Part model, mm, in its own coordinate system. A direction names the side the tool comes from. Give positions to 0.01 mm unless a question says otherwise; leave off trailing zeros. Write each loop counter-clockwise with the first axis right and the second up, starting at its lowest first coordinate (ties: lowest second). Pieces come first, ordered by that corner, then holes.
```python
from build123d import *

# Parameters (mm, degrees)
EXTRUDE_1_DEPTH     = 20
SKETCH_2_R          = 1.25
EXTRUDE_2_DEPTH     = 6
SKETCH_3_R          = 1.25
CUT_EXTRUDE_1_DEPTH = 6


with BuildPart() as part:
    # 草图1 → 凸台-拉伸1 (new body)
    with BuildSketch(Plane(origin=(0, 0, 0), x_dir=(1, 0, 0), z_dir=(0, 1, 0))):
        Polygon((2.125123473, -1.583145674), (2.433606108, 1.048838076), (0.308482635, 2.631983751), (-2.125123473, 1.583145674), (-2.433606108, -1.048838076), (-0.308482635, -2.631983751), align=None)
    extrude(amount=EXTRUDE_1_DEPTH)

    # 草图2 → 凸台-拉伸2 (add)
    with BuildSketch(Plane(origin=(0, 20, 0), x_dir=(1, 0, 0), z_dir=(0, 1, 0))):
        Circle(SKETCH_2_R)
    extrude(amount=EXTRUDE_2_DEPTH)

    # 草图3 → 切除-拉伸1 (cut)
    with BuildSketch(Plane.XZ):
        Circle(SKETCH_3_R)
    extrude(amount=-CUT_EXTRUDE_1_DEPTH, mode=Mode.SUBTRACT)


solid = part.part
```
1) Saw through at D-D, the plane z = 0. Write the cut outline in (x, y).
Answers follow:
outline: (-2.31, 0) - (-1.25, 0) - (-1.25, 6) - (1.25, 6) - (1.25, 0) - (2.31, 0) - (2.31, 20) - (1.25, 20) - (1.25, 26) - (-1.25, 26) - (-1.25, 20) - (-2.31, 20) - close
2) Saw through at A-A, the plane y = 3. Write the cut outline in (x, z), then the cut area to 3 significant figures.
Answers follow:
outline: (-2.43, 1.05) - (-2.13, -1.58) - (0.31, -2.63) - (2.43, -1.05) - (2.13, 1.58) - (-0.31, 2.63) - close; hole circle Ø2.5 at (0, 0)
area: 13.3 mm2
3) Two-plate mould, pull along Z, no slides. Class faces 1 (the face through (-0.27, 2.96, -1.22)), 2 (the face through (-1, 0, 1)), 3 (the face through (-0.27, 22.96, 1.22)): +Z half, -Z half, draft (parallel to the pull), parting line (faces both ways), or undercut.
Answers follow:
face 1: undercut
face 2: draft
face 3: parting line
4) Pin check, flat tips, straight feed: pin 1 Ø1.2 at (x, z) = (0, 0.5) entering from -Y; pin 2 Ø1.5 at (x, y) = (1, 14.5) entering from -Z; pin 3 Ø1.5 at (y, z) = (20.5, -1) entering from -X. Stop position of each tip, or through.
Answers follow:
pin 1: stops at y = 6
pin 2: stops at z = -2.63
pin 3: stops at x = -2.26
5) 3-axis set-ups, long thin cutter, end or side, ignore diameter. For faces 4 (the face through (0.891, 9.86, 2.115)), 5 (the face through (-1, 20, 1)), 6 (the face through (0, 6, 0)): which of +Z, -Z, +X, -X, +Y, -Y reach the whole face in a straight line?
Answers follow:
face 4: +Z, +X, +Y, -Y
face 5: +Y
face 6: -Y
6) Saw through at C-C, the plane x = 0.75. Write the cut outline in (y, z), then the cut area to 3 significant figures.
Answers follow:
outline: (0, -2.3) - (20, -2.3) - (20, -1) - (26, -1) - (26, 1) - (20, 1) - (20, 2.18) - (0, 2.18) - (0, 1) - (6, 1) - (6, -1) - (0, -1) - close
area: 89.6 mm2
7) Saw through at B-B, the plane y = 14.75. Write the cut outline in (x, z).
Answers follow:
outline: (-2.43, 1.05) - (-2.13, -1.58) - (0.31, -2.63) - (2.43, -1.05) - (2.13, 1.58) - (-0.31, 2.63) - close
8) Wall check: L1, parallel to Z at x = 0, y = 23.75; L2, parallel to Y at x = -0.5, z = -2.1; L3, parallel to Y at x = -1.15, z = -0.3. Give the ranges that are in metal, low to high.
Answers follow:
L1: z = -1.25 to 1.25
L2: y = 0 to 20
L3: y = 6 to 26
